Part model, mm, in its own coordinate system. A direction names the side the tool comes from. Round coordinates to 2 decimals unless told otherwise and drop trailing zeros. Loops run counter-clockwise (first coordinate to the right, second up) from the corner with the lowest first, then second, coordinate; pieces in that order, holes last.
1) Probe line 1 (X direction, y = 0.5, z = -24); line 2 (X direction, y = 3.5, z = -31.5); line 3 (Z direction, x = -38, y = 1.55). List the from-to ranges inside material, lowest first.
2) Band-saw the part on C-C, the plane z = -9.5. Write the cut outline in (x, y).
3) Band-saw the part on D-D, the plane x = -31.5. Write the cut outline in (y, z), then the cut area to 3 significant figures.
4) Band-saw the part on B-B, the plane y = 4.05. State how many separate pieces and enclosed holes the cut face has, then the cut area to 3 significant figures.
5) Band-saw the part on A-A, the plane y = 0.95. Write the cut outline in (x, z), then the cut area to 3 significant figures.
6) Mould opens along Z. For faces 4 (the flat face through (-39, 5, -22)), 5 (the cylindrical face through (-47.333, 4.037, -32.252)), 6 (the flat face through (-35, 2, -33.866)) say: +Z half, -Z half, draft (parallel to the pull), parting line (faces both ways), or undercut.
7) 3-axis set-ups, long thin cutter, end or side, ignore diameter. For faces 1 (the flat face through (-49.064, 1, -18)), 2 (the flat face through (-36, 0, -3)), 3 (the cylindrical face through (-36.44, 4.04, -31.03)): which of +Z, -Z, +X, -X, +Y, -Y reach the whole face in a straight line?
8) Drop a flat-ended pin along its axis: P1, Ø1, axis at x = -29, z = -26.5, coming from the -Y side. Give the stop position or say it passes through.
from build123d import *

# Parameters (mm, degrees)
SKETCH1_W           = 31.8
SKETCH1_H           = 31.8
BOSS_EXTRUDE1_DEPTH = 3.1
SKETCH2_W           = 28.8
SKETCH2_H           = 28.8
CUT_EXTRUDE1_DEPTH  = 1.9
SKETCH3_R           = 2.475
BOSS_EXTRUDE2_DEPTH = 1.9


with BuildPart() as part:
    # Sketch1 → Boss-Extrude1 (new body)
    with BuildSketch(Plane(origin=(0, 0, 0), x_dir=(1, 0, 0), z_dir=(0, 1, 0))):
        with Locations((-34.664493697, 17.966451592)):
            Rectangle(SKETCH1_W, SKETCH1_H)
    extrude(amount=BOSS_EXTRUDE1_DEPTH)

    # Sketch2 → Cut-Extrude1 (cut)
    with BuildSketch(Plane.XZ):
        with Locations((-34.664493697, -17.966451592)):
            Rectangle(SKETCH2_W, SKETCH2_H)
    extrude(amount=-CUT_EXTRUDE1_DEPTH, mode=Mode.SUBTRACT)

    # Sketch3 → Boss-Extrude2 (add)
    with BuildSketch(Plane(origin=(0, 3.1, 0), x_dir=(1, 0, 0), z_dir=(0, 1, 0))):
        with Locations(Location((-46.589493697, 29.891451592, 0), (0, 0, 90))):
            Circle(SKETCH3_R)
        with Locations(Location((-30.689493697, 29.891451592, 0), (0, 0, 90))):
            Circle(SKETCH3_R)
        with Locations(Location((-38.639493697, 29.891451592, 0), (0, 0, 90))):
            Circle(SKETCH3_R)
        with Locations(Location((-22.739493697, 29.891451592, 0), (0, 0, 90))):
            Circle(SKETCH3_R)
        with Locations(Location((-46.589493697, 21.941451592, 0), (0, 0, 90))):
            Circle(SKETCH3_R)
        with Locations(Location((-38.639493697, 21.941451592, 0), (0, 0, 90))):
            Circle(SKETCH3_R)
        with Locations(Location((-30.689493697, 21.941451592, 0), (0, 0, 90))):
            Circle(SKETCH3_R)
        with Locations(Location((-22.739493697, 21.941451592, 0), (0, 0, 90))):
            Circle(SKETCH3_R)
        with Locations(Location((-22.739493697, 13.991451592, 0), (0, 0, 90))):
            Circle(SKETCH3_R)
        with Locations(Location((-22.739493697, 6.041451592, 0), (0, 0, 90))):
            Circle(SKETCH3_R)
        with Locations(Location((-30.689493697, 13.991451592, 0), (0, 0, 90))):
            Circle(SKETCH3_R)
        with Locations(Location((-30.689493697, 6.041451592, 0), (0, 0, 90))):
            Circle(SKETCH3_R)
        with Locations(Location((-38.639493697, 13.991451592, 0), (0, 0, 90))):
            Circle(SKETCH3_R)
        with Locations(Location((-38.639493697, 6.041451592, 0), (0, 0, 90))):
            Circle(SKETCH3_R)
        with Locations(Location((-46.589493697, 13.991451592, 0), (0, 0, 90))):
            Circle(SKETCH3_R)
        with Locations(Location((-46.589493697, 6.041451592, 0), (0, 0, 90))):
            Circle(SKETCH3_R)
    extrude(amount=BOSS_EXTRUDE2_DEPTH)


solid = part.part
Reported:
1. line 1: x = -50.56 to -49.06, -20.26 to -18.76
1. line 2: x = -48.47 to -44.71, -40.52 to -36.76, -32.57 to -28.81, -24.62 to -20.86
1. line 3: z = -33.87 to -32.37, -3.57 to -2.07
2. outline: (-50.56, 0) - (-49.06, 0) - (-49.06, 1.9) - (-20.26, 1.9) - (-20.26, 0) - (-18.76, 0) - (-18.76, 3.1) - (-50.56, 3.1) - close
3. outline: (0, -33.87) - (3.1, -33.87) - (3.1, -32.23) - (5, -32.23) - (5, -27.55) - (3.1, -27.55) - (3.1, -24.28) - (5, -24.28) - (5, -19.6) - (3.1, -19.6) - (3.1, -16.33) - (5, -16.33) - (5, -11.65) - (3.1, -11.65) - (3.1, -8.38) - (5, -8.38) - (5, -3.7) - (3.1, -3.7) - (3.1, -2.07) - (0, -2.07) - (0, -3.57) - (1.9, -3.57) - (1.9, -32.37) - (0, -32.37) - close
3. area: 79.4 mm2
4. separate pieces: 16
4. enclosed holes: 0
4. area: 308 mm2
5. outline: (-50.56, -33.87) - (-18.76, -33.87) - (-18.76, -2.07) - (-50.56, -2.07) - close; hole (-49.06, -32.37) - (-20.26, -32.37) - (-20.26, -3.57) - (-49.06, -3.57) - close
5. area: 182 mm2
6. face 4: draft
6. face 5: undercut
6. face 6: -Z half
7. face 1: -Y
7. face 2: +Z, -Z, +X, -X, -Y
7. face 3: +Y
8. P1: stops at y = 1.9
